CAD build for the part. Positions are in the model's coordinates, mm. Coordinates: 2 decimals unless noted, no trailing zeros. Order: outer loops, then holes, each group sorted by start corner. A loop starts at its lowest first (then second) coordinate and runs counter-clockwise, first axis right, second up. Notation, with made-up numbers: (-6.5, -22) - (18.5, -22) arc R20 cw to (18.5, -12) - close; hole circle Ø4 at (61, 68.25). An arc over 180 degrees is marked (long way). Use one line per item in the form item = value.
```python
from build123d import *

# Parameters (mm, degrees)
F0_R            = 32.0294
F0_R_2          = 2.15265
F0_R_3          = 11.1125
F1_DEPTH        = 3.175
F3_DEPTH        = 3.175
F3_COPIES_COUNT = 4


# Not quite as in the source:
# - a pattern or mirror of a feature is missing from the dataset's text; its kind, count and spacing are read off the source's solid
# - a feature names something its author has since deleted; it is built from what else it names


with BuildPart() as f1:
    # F0 (on Top) → F1 (new body)
    with BuildSketch(Plane.XY):
        Circle(F0_R)
        with Locations((-11.7865861589, -11.7865861589)):
            Circle(F0_R_2, mode=Mode.SUBTRACT)
        with Locations((11.7865861589, -11.7865861589)):
            Circle(F0_R_2, mode=Mode.SUBTRACT)
        with Locations((-11.7865861589, 11.7865861589)):
            Circle(F0_R_2, mode=Mode.SUBTRACT)
        Circle(F0_R_3, mode=Mode.SUBTRACT)
        with Locations((11.7865861589, 11.7865861589)):
            Circle(F0_R_2, mode=Mode.SUBTRACT)
    extrude(amount=F1_DEPTH)

    # F2 (on face) → F3 (cut, through all)
    with BuildSketch(Plane.XY.offset(3.175)):
        with BuildLine():
            ThreePointArc((-11.229543123, 17.3148424047), (-8.0281867, 15.8788163052), (-6.3255746232, 12.8109235396))
            ThreePointArc((-6.3255746232, 12.8109235396), (0, 14.2875), (6.3255746232, 12.8109235396))
            ThreePointArc((6.3255746232, 12.8109235396), (8.0281867, 15.8788163052), (11.229543123, 17.3148424047))
            ThreePointArc((11.229543123, 17.3148424047), (0, 20.6375), (-11.229543123, 17.3148424047))
        make_face()
    f3 = extrude(amount=-F3_DEPTH, mode=Mode.SUBTRACT)

    # F3_copies: F3 ×4 about axis
    f3_copies_axis = Axis((0, 0, 0), (0, 0, 1))
    for i in range(1, F3_COPIES_COUNT):
        add(f3.rotate(f3_copies_axis, i * 360 / F3_COPIES_COUNT), mode=Mode.SUBTRACT)


solid = f1.part
```
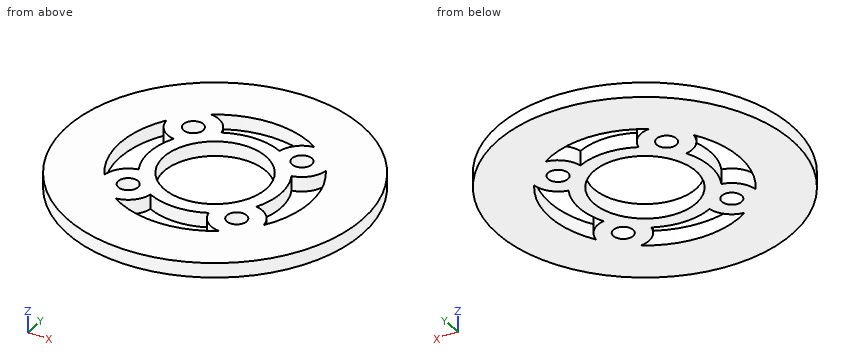
Item 1: Cut at A-A, the plane x = 0. Write the cut outline in (y, z) (1 decimal), plus the area to 3 significant figures.
Derived:
outline = (-32, 0) - (-20.6, 0) - (-20.6, 3.2) - (-32, 3.2) - close; (-14.3, 0) - (-11.1, 0) - (-11.1, 3.2) - (-14.3, 3.2) - close; (11.1, 0) - (14.3, 0) - (14.3, 3.2) - (11.1, 3.2) - close; (20.6, 0) - (32, 0) - (32, 3.2) - (20.6, 3.2) - close
area = 92.5 mm²
Item 2: Drill centre lines: line 1 (X direction, y = 0.5, z = 0.65); line 2 (Y direction, x = 0, z = 1.7); line 3 (Y direction, x = -4.5, z = 1.7). Where is each one in solid material? Low to high. Write a range as [from, to].
Derived:
line_1 = [-32.03, -20.63], [-14.28, -11.1], [11.1, 14.28], [20.63, 32.03]
line_2 = [-32.03, -20.64], [-14.29, -11.11], [11.11, 14.29], [20.64, 32.03]
line_3 = [-31.71, -20.14], [-13.56, -10.16], [10.16, 13.56], [20.14, 31.71]
Item 3: Cut at C-C, the plane x = 16. Write the cut outline in (y, z) (3 decimals), plus the area to 3 significant figures.
Derived:
outline = (-27.747, 0) - (-8.165, 0) - (-8.165, 3.175) - (-27.747, 3.175) - close; (8.165, 0) - (27.747, 0) - (27.747, 3.175) - (8.165, 3.175) - close
area = 124 mm²
Item 4: Cut at D-D, the plane z = 0.5. State how many separate pieces and enclosed holes the cut face has, plus the area to 3 significant figures.
Derived:
separate_pieces = 1
enclosed_holes = 9
area = 2,350 mm²
Item 5: Drop flat-ended pins along their axis: pin 1 (1.5 mm diameter, centred on x = -6.5, z = 2, fed in from -Y); pin 2 (1 mm diameter, centred on y = 25.5, z = 0.5, fed in from +X); pin 3 (3.5 mm diameter, centred on x = 11.79, y = 11.79, fed in from -Z); pin 4 (1 mm diameter, centred on x = -11.5, y = -1.5, fed in from -Z). Give the stop position or say it passes through.
Derived:
pin_1 = -31.51
pin_2 = 20.02
pin_3 = through
pin_4 = 0
